Verification items for the finished model (mm, model axes). Give positions to 0.01 mm unless a question says otherwise; leave off trailing zeros. Order: outer loops, then holes, each group sorted by start corner. A loop starts at its lowest first (then second) coordinate and runs counter-clockwise, first axis right, second up. Notation, with made-up numbers: (8, 87) - (13, 87) arc R14 cw to (13, 103) - close; hole circle Ø4 at (48.5, -25.5). An arc over 180 degrees is marked (long way). Answer as a JSON object with one key per item and string values.
```python
from build123d import *

# Parameters (mm, degrees)
SKETCH_1_W      = 400
SKETCH_1_H      = 200
EXTRUDE_1_DEPTH = 3


with BuildPart() as part:
    # 草图1 → 凸台-拉伸1 (new body)
    with BuildSketch(Plane(origin=(0, 0, 0), x_dir=(1, 0, 0), z_dir=(0, 1, 0))):
        with BuildLine():
            Line((2, 0), (758, 0))
            ThreePointArc((758, 0), (759.414213562, 0.585786438), (760, 2))
            Line((760, 2), (760, 210))
            ThreePointArc((760, 210), (759.414213562, 211.414213562), (758, 212))
            Line((758, 212), (2, 212))
            ThreePointArc((2, 212), (0.585786438, 211.414213562), (0, 210))
            Line((0, 210), (0, 2))
            ThreePointArc((0, 2), (0.585786438, 0.585786438), (2, 0))
        make_face()
        with Locations((380, 106)):
            Rectangle(SKETCH_1_W, SKETCH_1_H, mode=Mode.SUBTRACT)
        with BuildLine():
            Line((658, 6), (602, 6))
            ThreePointArc((602, 6), (600.585786438, 6.585786438), (600, 8))
            Line((600, 8), (600, 204))
            ThreePointArc((600, 204), (600.585786438, 205.414213562), (602, 206))
            Line((602, 206), (658, 206))
            ThreePointArc((658, 206), (659.414213562, 205.414213562), (660, 204))
            Line((660, 204), (660, 8))
            ThreePointArc((660, 8), (659.414213562, 6.585786438), (658, 6))
        make_face(mode=Mode.SUBTRACT)
        with BuildLine():
            Line((158, 6), (102, 6))
            ThreePointArc((102, 6), (100.585786438, 6.585786438), (100, 8))
            Line((100, 8), (100, 204))
            ThreePointArc((100, 204), (100.585786438, 205.414213562), (102, 206))
            Line((102, 206), (158, 206))
            ThreePointArc((158, 206), (159.414213562, 205.414213562), (160, 204))
            Line((160, 204), (160, 8))
            ThreePointArc((160, 8), (159.414213562, 6.585786438), (158, 6))
        make_face(mode=Mode.SUBTRACT)
        with BuildLine():
            Line((38, 160), (22, 160))
            ThreePointArc((22, 160), (20.585786438, 160.585786438), (20, 162))
            Line((20, 162), (20, 178))
            ThreePointArc((20, 178), (20.585786438, 179.414213562), (22, 180))
            Line((22, 180), (38, 180))
            ThreePointArc((38, 180), (39.414213562, 179.414213562), (40, 178))
            Line((40, 178), (40, 162))
            ThreePointArc((40, 162), (39.414213562, 160.585786438), (38, 160))
        make_face(mode=Mode.SUBTRACT)
        with BuildLine():
            Line((718, 160), (702, 160))
            ThreePointArc((702, 160), (700.585786438, 160.585786438), (700, 162))
            Line((700, 162), (700, 178))
            ThreePointArc((700, 178), (700.585786438, 179.414213562), (702, 180))
            Line((702, 180), (718, 180))
            ThreePointArc((718, 180), (719.414213562, 179.414213562), (720, 178))
            Line((720, 178), (720, 162))
            ThreePointArc((720, 162), (719.414213562, 160.585786438), (718, 160))
        make_face(mode=Mode.SUBTRACT)
    extrude(amount=-EXTRUDE_1_DEPTH)


solid = part.part
```
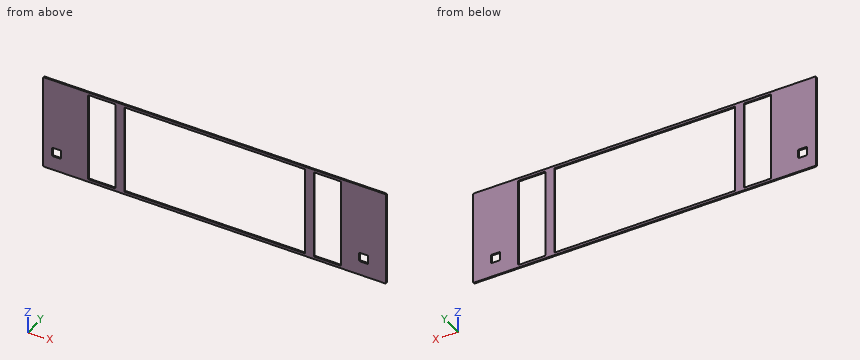
(1) Section check B-B (z = -117). Record the cut outline in (x, y).
Computed values:
{"outline": "(0, -3) - (100, -3) - (100, 0) - (0, 0) - close; (160, -3) - (180, -3) - (180, 0) - (160, 0) - close; (580, -3) - (600, -3) - (600, 0) - (580, 0) - close; (660, -3) - (760, -3) - (760, 0) - (660, 0) - close"}
(2) Section check C-C (y = -1.55). Count the separate pieces of the cut face and the enclosed holes in it, then the cut area to 3 significant figures.
Computed values:
{"separate pieces": "1", "enclosed holes": "5", "area": "56,300 mm²"}
(3) Section check A-A (x = 396.5). Record the cut outline in (y, z).
Computed values:
{"outline": "(-3, -212) - (0, -212) - (0, -206) - (-3, -206) - close; (-3, -6) - (0, -6) - (0, 0) - (-3, 0) - close"}
(4) Material ranges on line 1 along X through (y, z) = (-2.5, -185); line 2 along X through (y, z) = (-1.95, -166); line 3 along Z through (x, y) = (305, -1.9), recorded low to high. Write a range as [from, to].
Computed values:
{"line 1": "x = [0, 100], [160, 180], [580, 600], [660, 760]", "line 2": "x = [0, 20], [40, 100], [160, 180], [580, 600], [660, 700], [720, 760]", "line 3": "z = [-212, -206], [-6, 0]"}
